Source: CAD feature listing. Evaluate the final solid. Frame: model axes, mm. A direction names the side the tool comes from. Give positions to 0.01 mm unless a question says otherwise; leave off trailing zeros. Loops run counter-clockwise (first coordinate to the right, second up) from the corner with the lowest first, then second, coordinate; pieces in that order, holes last. Notation, with made-up numbers: M 43.5,18 L 68.5,18 A23 ccw 68.5,34 Z; hole C -38.75,47.5 d5. An arc over 180 degrees is marked long. Write item = value, one per line.
from build123d import *

# Parameters (mm, degrees)
F1_DEPTH = 25.4
F3_DEPTH = 25.4


with BuildPart() as f1:
    # F0 (on Front) → F1 (new body)
    with BuildSketch(Plane.XZ):
        Polygon((-12.7, 0), (0, 0), (25.4, 0), (25.4, 31.75), (-12.7, 31.75), align=None)
    extrude(amount=F1_DEPTH)

    # F2 (on face) → F3 (cut)
    with BuildSketch(Plane.YZ.offset(25.4)):
        Polygon((-25.4, 31.75), (-25.4, 6.35), (0, 31.75), align=None)
    extrude(amount=-F3_DEPTH, mode=Mode.SUBTRACT)


solid = f1.part
1. Cut plane A-A, the plane z = 25. Return the cut outline in (x, y).
Derived:
outline = M -12.7,-25.4 L 0,-25.4 L 0,-6.75 L 25.4,-6.75 L 25.4,0 L -12.7,0 Z
2. Material intervals for probe 1 along X at (y, z) = (-15.5, 21); probe 2 along Y at (x, z) = (15, 20); probe 3 along Y at (x, z) = (20.5, 27), sorted ascending. Write a range as from..to.
Derived:
probe_1 = -12.7..0
probe_2 = -11.75..0
probe_3 = -4.75..0
3. Reachability of faces 1 (the flat face through (6, 0, 16)), 2 (the flat face through (0, -16, 22)) from +Z, -Z, +X, -X, +Y, -Y: full face, straight path, thin tool, end or side. Return the list, or none.
Derived:
face_1 = +Z, -Z, +X, -X, +Y
face_2 = +Z, +X, -Y
4. First-contact query: pin 1 Ø10 at (x, y) = (4, -22.5) entering from +Z; pin 2 Ø7.5 at (y, z) = (-15, 25.5) entering from +X; pin 3 Ø6 at (x, y) = (9, -5.5) entering from +Z. Flat tips, straight axial feed; report the tip coordinate or a pass-through.
Derived:
pin_1 = 31.75
pin_2 = 0
pin_3 = 29.25
5. Cut plane B-B, the plane y = -13.5. Return the cut outline in (x, z), then the cut area to 3 significant figures.
Derived:
outline = M -12.7,0 L 25.4,0 L 25.4,18.25 L 0,18.25 L 0,31.75 L -12.7,31.75 Z
area = 867 mm²
6. Cut plane C-C, the plane x = 19.5. Return the cut outline in (y, z).
Derived:
outline = M -25.4,0 L 0,0 L 0,31.75 L -25.4,6.35 Z
